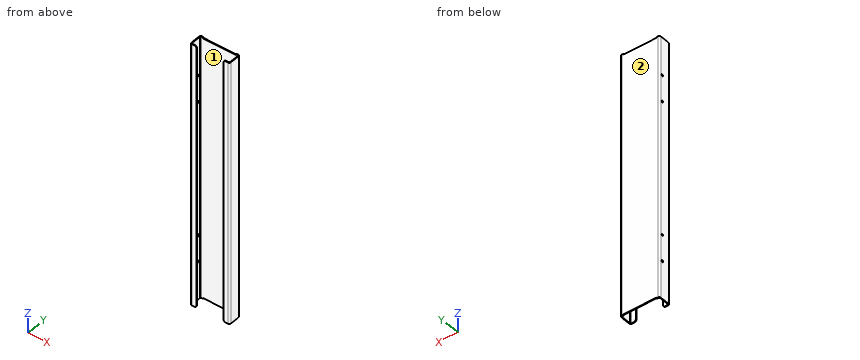
```python
from build123d import *

# Parameters (mm, degrees)
BASE_FLANGE1_DEPTH = 347
SKETCH4_W          = 87
SKETCH4_H          = 2
CUT_EXTRUDE1_DEPTH = 10
SKETCH8_R          = 2.5
CUT_EXTRUDE5_DEPTH = 10
LPATTERN4_COUNT    = 2
LPATTERN4_PITCH    = 424
FILLET1_R          = 5


# Sheet-metal steps are written as plain solids
with BuildPart() as part:
    # Sketch3 → Base-Flange1 (new, symmetric)
    with BuildSketch(Plane.XY):
        with BuildLine():
            Line((36, -33), (48, -33))
            ThreePointArc((48, -33), (50.828427125, -31.828427125), (52, -29))
            Line((52, -29), (52, -4))
            ThreePointArc((52, -4), (50.828427125, -1.171572875), (48, 0))
            Line((48, 0), (-48, 0))
            ThreePointArc((-48, 0), (-50.828427125, -1.171572875), (-52, -4))
            Line((-52, -4), (-52, -29))
            ThreePointArc((-52, -29), (-50.828427125, -31.828427125), (-48, -33))
            Line((-48, -33), (-36, -33))
            Line((-36, -33), (-36, -31))
            Line((-36, -31), (-48, -31))
            ThreePointArc((-48, -31), (-49.414213562, -30.414213562), (-50, -29))
            Line((-50, -29), (-50, -4))
            ThreePointArc((-50, -4), (-49.414213562, -2.585786438), (-48, -2))
            Line((-48, -2), (48, -2))
            ThreePointArc((48, -2), (49.414213562, -2.585786438), (50, -4))
            Line((50, -4), (50, -29))
            ThreePointArc((50, -29), (49.414213562, -30.414213562), (48, -31))
            Line((48, -31), (36, -31))
            Line((36, -31), (36, -33))
        make_face()
    extrude(amount=BASE_FLANGE1_DEPTH, both=True)

    # Sketch4 → Cut-Extrude1 (cut)
    with BuildSketch(Plane(origin=(0, 0, 0), x_dir=(1, 0, 0), z_dir=(0, 1, 0))):
        with Locations((0, -346)):
            Rectangle(SKETCH4_W, SKETCH4_H)
        with Locations((0, 346)):
            Rectangle(SKETCH4_W, SKETCH4_H)
    extrude(amount=-CUT_EXTRUDE1_DEPTH, mode=Mode.SUBTRACT)

    # Sketch8 → Cut-Extrude5 (cut)
    with BuildSketch(Plane.ZY.offset(52)):
        with Locations(Location((177, -9, 0), (0, 0, 270))):
            Circle(SKETCH8_R)
        with Locations(Location((247, -9, 0), (0, 0, 270))):
            Circle(SKETCH8_R)
    cut_extrude5 = extrude(amount=-CUT_EXTRUDE5_DEPTH, mode=Mode.SUBTRACT)

    # LPattern4: Cut-Extrude5 ×2
    with Locations(*[(0, 0, -i * LPATTERN4_PITCH) for i in range(1, LPATTERN4_COUNT)]):
        add(cut_extrude5, mode=Mode.SUBTRACT)

    # Fillet1
    fillet1_edges = [part.edges().sort_by_distance(p)[0] for p in [
        (-36, -32, -347),
        (36, -32, -347),
        (-36, -32, 347),
        (36, -32, 347),
    ]]
    fillet(fillet1_edges, radius=FILLET1_R)


solid = part.part
```
Model file for the job. Use its own axes, mm. Face numbers are marked on the shaded views. Give positions to 0.01 mm unless a question says otherwise; leave off trailing zeros. Loops run counter-clockwise (first coordinate to the right, second up) from the corner with the lowest first, then second, coordinate; pieces in that order, holes last. Notation, with made-up numbers: (1.5, -10.75) - (43.5, -10.75) arc R25 ccw to (43.5, 24.25) - close; hole circle Ø2 at (-8.75, 71). An arc over 180 degrees is marked (long way). One line per item, written item: value. Start each with the question number.
1. Slice it at C-C (x = 19). List the corners of the cut face in (y, z), plus the area to 3 significant figures.
2. Probe L1, parallel to Z at x = -51.05, y = -9; L2, parallel to Y at x = -51.4, z = 247; L3, parallel to X at y = -6, z = 259. List the from-to ranges inside material, lowest first. Write a range as from..to.
3. Pull direction Y, two halves, no side cores. Call the marked faces 1 and 2: pulls with the +Y half, pulls with the -Y half, needs draft (parallel to the pull), parting line crosses it, or undercut.
4. Slice it at A-A (y = -19.5). List the corners of the cut face in (x, z), plus the area to 3 significant figures.
5. Slice it at B-B (z = -72.5). List the corners of the cut face in (x, y).
6. Pin check, flat tips, straight feed: pin 1 (1.6 mm diameter, centred on y = -0.5, z = -345.5, fed in from +X); pin 2 (0.6 mm diameter, centred on y = -32, z = -68, fed in from -X); pin 3 (1 mm diameter, centred on y = -31.5, z = 116.5, fed in from +X). Stop position of each tip, or through.
Solution:
1. outline: (-2, -345) - (0, -345) - (0, 345) - (-2, 345) - close
1. area: 1,380 mm^2
2. L1: z = -347..-249.5, -244.5..-179.5, -174.5..174.5, 179.5..244.5, 249.5..347
2. L2: y = -31.11..-11.5, -6.5..-1.89
2. L3: x = -52..-50, 50..52
3. face 1: undercut
3. face 2: pulls with the +Y half
4. outline: (-52, -347) - (-50, -347) - (-50, 347) - (-52, 347) - close; (50, -347) - (52, -347) - (52, 347) - (50, 347) - close
4. area: 2,780 mm^2
5. outline: (-52, -29) arc R4 ccw to (-48, -33) - (-36, -33) - (-36, -31) - (-48, -31) arc R2 cw to (-50, -29) - (-50, -4) arc R2 cw to (-48, -2) - (48, -2) arc R2 cw to (50, -4) - (50, -29) arc R2 cw to (48, -31) - (36, -31) - (36, -33) - (48, -33) arc R4 ccw to (52, -29) - (52, -4) arc R4 ccw to (48, 0) - (-48, 0) arc R4 ccw to (-52, -4) - close
6. pin 1: stops at x = 50.95
6. pin 2: stops at x = -50.95
6. pin 3: stops at x = 51.46
